Check sheet for the modelled part. Datum: model origin and axes. Units: mm. A direction names the side the tool comes from. Round coordinates to 2 decimals unless told otherwise and drop trailing zeros. Write each loop counter-clockwise with the first axis right and the second up, starting at its lowest first coordinate (ties: lowest second). Pieces come first, ordered by that corner, then holes. Notation, with made-up numbers: (-27, 62.25) -> (26, 62.25) arc R16 cw to (26, 86.25) -> close; hole circle Ø8 at (-28, 76.25). An arc over 180 degrees is marked (long way). One line per item, written item: value. Start each with the question number.
```python
from build123d import *

# Parameters (mm, degrees)
BOSS_EXTRUDE1_DEPTH  = 5
CUT_EXTRUDE1_DEPTH   = 5
SKETCH6_R            = 1
BOSS_EXTRUDE5_DEPTH  = 1.25
SKETCH7_R            = 1
BOSS_EXTRUDE6_DEPTH  = 1.25
SKETCH8_R            = 1
BOSS_EXTRUDE7_DEPTH  = 1.25
BOSS_EXTRUDE8_START  = 1.25
SKETCH9_R            = 1
BOSS_EXTRUDE8_DEPTH  = 1.25
SKETCH10_R           = 1
BOSS_EXTRUDE12_DEPTH = 1.25
BOSS_EXTRUDE13_START = 1.25
SKETCH11_R           = 1
BOSS_EXTRUDE13_DEPTH = 1.25
BOSS_EXTRUDE14_START = 1.25
SKETCH12_R           = 1
BOSS_EXTRUDE14_DEPTH = 1.25


with BuildPart() as part:
    # Sketch3 → Boss-Extrude1 (new body)
    with BuildSketch(Plane(origin=(0, 0, 0), x_dir=(1, 0, 0), z_dir=(0, 1, 0))):
        Polygon((41, 0), (28.991378029, 28.991378029), (0, 41), (-28.991378029, 28.991378029), (-41, 0), (-28.991378029, -28.991378029), (0, -41), (28.991378029, -28.991378029), align=None)
    extrude(amount=BOSS_EXTRUDE1_DEPTH)

    # Sketch5 → Cut-Extrude1 (cut)
    with BuildSketch(Plane(origin=(0, 5, 0), x_dir=(1, 0, 0), z_dir=(0, 1, 0))):
        Polygon((35.75, 0), (25.279067427, 25.279067427), (0, 35.75), (-25.279067427, 25.279067427), (-35.75, 0), (-25.279067427, -25.279067427), (0, -35.75), (25.279067427, -25.279067427), align=None)
    extrude(amount=-CUT_EXTRUDE1_DEPTH, mode=Mode.SUBTRACT)

    # Sketch6 → Boss-Extrude5 (add)
    with BuildSketch(Plane(origin=(14.495689014, 0, 34.995689014), x_dir=(0.9238795325112827, 0, -0.38268343236509966), z_dir=(0.38268343236509966, 0, 0.9238795325112827))):
        with Locations(Location((0, 3, 0), (0, 0, 180))):
            Circle(SKETCH6_R)
        with Locations(Location((-5, 3, 0), (0, 0, 180))):
            Circle(SKETCH6_R)
        with Locations(Location((5, 3, 0), (0, 0, 180))):
            Circle(SKETCH6_R)
    extrude(amount=BOSS_EXTRUDE5_DEPTH)

    # Sketch7 → Boss-Extrude6 (add)
    with BuildSketch(Plane(origin=(-34.995689014, 0, 14.495689014), x_dir=(0.3826834323650997, 0, 0.9238795325112827), z_dir=(-0.9238795325112827, 0, 0.3826834323650997))):
        with Locations(Location((5, 3, 0), (0, 0, 180))):
            Circle(SKETCH7_R)
    extrude(amount=BOSS_EXTRUDE6_DEPTH)

    # Sketch8 → Boss-Extrude7 (add)
    with BuildSketch(Plane(origin=(-34.995689014, 0, -14.495689014), x_dir=(-0.3826834323650795, 0, 0.9238795325112911), z_dir=(-0.9238795325112911, 0, -0.3826834323650795))):
        with Locations(Location((0, 3, 0), (0, 0, 180))):
            Circle(SKETCH8_R)
    extrude(amount=BOSS_EXTRUDE7_DEPTH)

    # Sketch9 → Boss-Extrude8 (add)
    with BuildSketch(Plane(origin=(-14.495689014, 0, -34.995689014), x_dir=(-0.9238795325112826, 0, 0.38268343236509983), z_dir=(-0.38268343236509983, 0, -0.9238795325112826)).offset(BOSS_EXTRUDE8_START)):
        with Locations((-5, 3)):
            Circle(SKETCH9_R)
    extrude(amount=-BOSS_EXTRUDE8_DEPTH)

    # Sketch10 → Boss-Extrude12 (add)
    with BuildSketch(Plane(origin=(14.495689014, 0, -34.995689014), x_dir=(-0.923879532511291, 0, -0.38268343236507973), z_dir=(0.38268343236507973, 0, -0.923879532511291))):
        with Locations(Location((0, 3, 0), (0, 0, 180))):
            Circle(SKETCH10_R)
        with Locations(Location((5, 3, 0), (0, 0, 180))):
            Circle(SKETCH10_R)
    extrude(amount=BOSS_EXTRUDE12_DEPTH)

    # Sketch11 → Boss-Extrude13 (add)
    with BuildSketch(Plane(origin=(34.995689014, 0, -14.495689014), x_dir=(-0.3826834323651001, 0, -0.9238795325112825), z_dir=(0.9238795325112824, 0, -0.38268343236510005)).offset(BOSS_EXTRUDE13_START)):
        with Locations(Location((5, 3, 0), (0, 0, 180))):
            Circle(SKETCH11_R)
        with Locations((-5, 3)):
            Circle(SKETCH11_R)
    extrude(amount=-BOSS_EXTRUDE13_DEPTH)

    # Sketch12 → Boss-Extrude14 (add)
    with BuildSketch(Plane(origin=(34.995689014, 0, 14.495689014), x_dir=(0.3826834323650795, 0, -0.923879532511291), z_dir=(0.9238795325112911, 0, 0.38268343236507957)).offset(BOSS_EXTRUDE14_START)):
        with Locations((0, 3)):
            Circle(SKETCH12_R)
        with Locations(Location((-5, 3, 0), (0, 0, 180))):
            Circle(SKETCH12_R)
    extrude(amount=-BOSS_EXTRUDE14_DEPTH)


solid = part.part
```
1. Cross-section at B-B (x = -31). Record the cut outline in (y, z).
2. Material ranges on probe 1 along Z at (x, y) = (34, 2.1); probe 2 along X at (y, z) = (3.85, -21.5); probe 3 along X at (y, z) = (2.8, 24), recorded low to high.
3. Cross-section at A-A (z = 28). Record the cut outline in (x, y), plus the area to 3 significant figures.
4. Depth check by flat-ended pin: pin 1 Ø1 at (y, z) = (3.5, -22) entering from -X; pin 2 Ø3 at (y, z) = (1.5, 29.5) entering from -X; pin 3 Ø3 at (x, y) = (-32, 3.5) entering from -Z. Enter the tip coordinate at first touch or a pass-through.
5. Release check for a two-part mould opening along X. For faces 3 (the face through (34.02, 3.38, -18.5)), 4 (the face through (15, 5, 30)), 5 (the face through (38.07, 3.01, -10.34)) record: +X half, -X half, draft (parallel to the pull), parting line (faces both ways), or undercut.
6. Access from +Z, -Z, +X, -X, +Y, -Y to the whole of each face (thin tool, end or side, straight path). Record for faces 1 (the face through (10.845, 3.608, 37.175)), 2 (the face through (12.46, 2.54, 30.59)).
Working result:
1. outline: (0, -24.14) -> (5, -24.14) -> (5, -11.47) -> (0, -11.47) -> close; (0, 11.47) -> (5, 11.47) -> (5, 24.14) -> (0, 24.14) -> close
2. probe 1: z = -19.97 to -19.02, -16.9 to -4.22, 4.22 to 16.9, 19.02 to 19.97
2. probe 2: x = -32.09 to -26.84, 26.84 to 32.09
2. probe 3: x = -31.06 to -25.81, 25.81 to 31.06
3. outline: (-29.4, 0) -> (-18.71, 0) -> (-18.71, 5) -> (-29.4, 5) -> close; (18.71, 0) -> (29.4, 0) -> (29.4, 5) -> (18.71, 5) -> close
3. area: 107 mm^2
4. pin 1: stops at x = -32.09
4. pin 2: stops at x = -29.4
4. pin 3: stops at z = -25.35
5. face 3: undercut
5. face 4: draft
5. face 5: +X half
6. face 1: none
6. face 2: +Y, -Y
